The model under review builds one solid part; all positions refer to its coordinate system, in mm. Coordinates: 2 decimals unless noted, no trailing zeros. Order: outer loops, then holes, each group sorted by start corner. A loop starts at its lowest first (then second) coordinate and runs counter-clockwise, first axis right, second up. Notation, with made-up numbers: M 42,-9 L 90,-9 A36 ccw 90,28 Z; hole C 81.25,50 d2. An arc over 180 degrees is marked long. Answer as CSV lines item,"result". Start each with the question number.
Q1. For P1, Ø24, axis at y = -88, z = -58, coming from the +X side, flat-tipped, find the tip position at first contact; note if it passes through.
Q2. Consider section D-D on z = -58. Write out the cut boundary in (x, y).
Q3. The part is to be moulded in two halves that separate along Z. For faces 1 (the face through (3, -2, -115)), 2 (the face through (3, 0, -59)), 3 (the face through (2.788, -102.643, -54.748)), 4 (the face through (3, -54, 0)), say which applies: +Z half, -Z half, draft (parallel to the pull), parting line (faces both ways), or undercut.
Q4. Wall thickness on L1, parallel to Y at x = 2, z = -58; L2, parallel to Y at x = 3.2, z = -7.5; L3, parallel to Z at x = 3.65, y = -5: over which ranges is each line inside the solid? List them lowest first. Write a range as [from, to].
Q5. Consider section C-C on z = -108.5. Write out the cut boundary in (x, y).
Q6. Consider section B-B on x = 4.55. Write out the cut boundary in (y, z), and give its area (3 significant figures).
Q7. Consider section A-A on y = -10. Write out the cut boundary in (x, z).
Autodesk Inventor part; units mm, degrees
ref_plane "YZ Plane" through (0, 0, 0) normal (1, 0, 0) x (0, 1, 0)
ref_plane "XZ Plane" through (0, 0, 0) normal (0, 1, 0) x (-1, 0, 0)
ref_plane "XY Plane" through (0, 0, 0) normal (0, 0, 1) x (1, 0, 0)
sketch "スケッチ1" plane through (0, 0, 0) normal (1, 0, 0) x (0, 1, 0)
  line L0 (0, 0) -> (-110, 0)
  line L1 (-110, 0) -> (-110, -116)
  line L2 (-110, -116) -> (0, -116)
  line L3 (0, -116) -> (0, 0)
  dimension "d0" = 110
  dimension "d1" = 116
extrude "押し出し1" add sketch "スケッチ1" along normal blind 5.5
fillet "フィレット1" radius 5 4 edges at (2.75, 0, 0) (2.75, 0, -116) (2.75, -110, 0) (2.75, -110, -116)
sketch "スケッチ2" plane through (5.5, 0, 0) normal (1, 0, 0) x (0, 0, -1)
  line L0 (7.5, -5) -> (108.5, -5)
  line L1 (108.5, -5) -> (108.5, -105)
  line L2 (108.5, -105) -> (7.5, -105)
  line L3 (7.5, -105) -> (7.5, -5)
  line L4 (111, 0) -> (5, 0)
  line L5 (0, -5) -> (0, -105)
  point P0 (0, 0)
  dimension "d5" = 101
  dimension "d6" = 100
  dimension "d7" = 5
  dimension "d8" = 7.5
hole "穴1" at (5.5, -5, -7.5) at (5.5, -5, -108.5) at (5.5, -105, -108.5) at (5.5, -105, -7.5) direction (-1, 0, 0) diameter 3 end through all
sketch "スケッチ3" plane through (5.5, 0, 0) normal (1, 0, 0) x (0, 0, -1)
  circle A0 centre (58, -88) radius 15
  line L0 (0, -5) -> (0, -105)
  line L1 (5, -110) -> (111, -110)
  point P0 (0, 0)
  dimension "d16" = 30
  dimension "d17" = 58
  dimension "d18" = 22
extrude "押し出し2" cut sketch "スケッチ3" against normal through all
sketch "スケッチ4" plane through (5.5, 0, 0) normal (1, 0, 0) x (0, 0, -1)
  circle A0 centre (58, -22) radius 15
  line L0 (111, 0) -> (5, 0)
  circle A1 centre (58, -88) radius 15
  line L1 (0, -5) -> (0, -105)
  point P0 (0, 0)
  dimension "d21" = 30
  dimension "d22" = 22
  dimension "d23" = 58
  dimension "d24" = 58
sketch "スケッチ5" plane through (5.5, 0, 0) normal (1, 0, 0) x (0, 0, -1)
  point P0 (0, 0)
extrude "押し出し3" cut sketch "スケッチ4" against normal through all contours A0
equation "\"d24\" = d23"
properties part number "ロボットベースT5.5_2" material "木材 (オーク)"
Evaluation:
1,P1,"passes through"
2,outline,"M 0,-110 L 5.5,-110 L 5.5,-103 L 0,-103 Z; M 0,-73 L 5.5,-73 L 5.5,-37 L 0,-37 Z; M 0,-7 L 5.5,-7 L 5.5,0 L 0,0 Z"
3,face 1,"-Z half"
3,face 2,"draft"
3,face 3,"undercut"
3,face 4,"+Z half"
4,L1,"y = [-110, -103], [-73, -37], [-7, 0]"
4,L2,"y = [-110, -106.5], [-103.5, -6.5], [-3.5, 0]"
4,L3,"z = [-116, -110], [-107, -9], [-6, 0]"
5,outline,"M 0,-110 L 5.5,-110 L 5.5,-106.5 L 0,-106.5 Z; M 0,-103.5 L 5.5,-103.5 L 5.5,-6.5 L 0,-6.5 Z; M 0,-3.5 L 5.5,-3.5 L 5.5,0 L 0,0 Z"
6,outline,"M -110,-111 A5 ccw -105,-116 L -5,-116 A5 ccw 0,-111 L 0,-5 A5 ccw -5,0 L -105,0 A5 ccw -110,-5 Z; hole C -105,-108.5 d3; hole C -105,-7.5 d3; hole C -88,-58 d30; hole C -22,-58 d30; hole C -5,-108.5 d3; hole C -5,-7.5 d3"
6,area,"11,300 mm²"
7,outline,"M 0,-116 L 5.5,-116 L 5.5,-67 L 0,-67 Z; M 0,-49 L 5.5,-49 L 5.5,0 L 0,0 Z"
